```python
from build123d import *

# Parameters (mm, degrees)
F0_R          = 6
F1_DEPTH      = 30
F1_DEPTH_BACK = 30


# Not quite as in the source:
# - a pattern or mirror of a feature is missing from the dataset's text; its kind, count and spacing are read off the source's solid


with BuildPart() as f1:
    # F0 (on Front) → F1 (new body, two sides)
    with BuildSketch(Plane.XZ) as f1_sk:
        Circle(F0_R)
    extrude(amount=F1_DEPTH)
    extrude(f1_sk.sketch, amount=-F1_DEPTH_BACK)

    # F2 (on Right) → F3 (revolve)
    with BuildSketch(Plane.YZ):
        with BuildLine():
            Line((-31.8, 0), (-30, 0))
            Line((-30, 0), (-30, 6))
            ThreePointArc((-30, 6), (-31.3403065089, 3.1320919527), (-31.8, 0))
        make_face()
    f3 = revolve(axis=Axis((0, 0, 0), (0, 1, 0)))

    # F3_copies: F3 across plane
    add(f3.mirror(Plane.ZX))


solid = f1.part
```
Source: CAD feature listing. Evaluate the final solid. Frame: model axes, mm. Coordinates: 2 decimals unless noted, no trailing zeros. Loops run counter-clockwise (first coordinate to the right, second up) from the corner with the lowest first, then second, coordinate; pieces in that order, holes last. Notation, with made-up numbers: (-31, 36.5) -> (4, 36.5) arc R21 ccw to (4, 66.5) -> close; hole circle Ø9 at (43.25, -24.75). An arc over 180 degrees is marked (long way). One line per item, written item: value. Start each with the question number.
Q1. Line query: line 1 along X through (y, z) = (16.5, 3.5); line 2 along Y through (x, z) = (4.25, -3.5); line 3 along Z through (x, y) = (-1.5, 14.5). Output: solid intervals per line, ascending.
Q2. Section query C-C, the plane z = 0. Return the cut outline in (x, y), and give its area (3 significant figures).
Q3. Section query A-A, the plane x = 0. Return the cut outline in (y, z), and give its area (3 significant figures).
Q4. Section query B-B, the plane y = -19.5. Return the cut outline in (x, z).
Q5. Contact query for flat-ended pins moving along their axis: P1, Ø2, axis at x = -2, z = -2, coming from the -Y side; P2, Ø6, axis at x = -4.5, z = -0.5, coming from the -Y side; P3, Ø1, axis at y = 17.5, z = -4.5, coming from the +X side. Output: stop coordinate, or through.
Results:
1. line 1: -4.87 to 4.87
1. line 2: -30.31 to 30.31
1. line 3: -5.81 to 5.81
2. outline: (-6, -30) arc R10.9 ccw to (6, -30) -> (6, 30) arc R10.9 ccw to (-6, 30) -> close
2. area: 749 mm^2
3. outline: (-30, -6) -> (30, -6) arc R10.9 ccw to (30, 6) -> (-30, 6) arc R10.9 ccw to start
3. area: 749 mm^2
4. outline: circle Ø12 at (0, 0)
5. P1: y = -31.65
5. P2: y = -31.69
5. P3: x = 4.47
